from build123d import *

# Parameters (mm, degrees)
SKETCH1_W           = 225.425
SKETCH1_H           = 196.85
SKETCH1_R           = 2.5527
BOSS_EXTRUDE1_DEPTH = 3.175
FILLET1_R           = 6.35
SKETCH2_W           = 22.86
SKETCH2_H           = 31.75
CUT_EXTRUDE1_DEPTH  = 300.293223695
FILLET2_R           = 6.35
BOSS_EXTRUDE2_DEPTH = 3.175
FILLET3_R           = 6.35
SKETCH4_R           = 2.4892
CUT_EXTRUDE2_DEPTH  = 520.25515638
CUT_EXTRUDE3_DEPTH  = 520.25515638
FILLET4_R           = 12.7
FILLET5_R           = 12.7
CUT_EXTRUDE4_DEPTH  = 520.25515638
FILLET6_R           = 12.7


with BuildPart() as part:
    # Sketch1 → Boss-Extrude1 (new body)
    with BuildSketch(Plane(origin=(0, 0, 0), x_dir=(1, 0, 0), z_dir=(0, 1, 0))):
        with Locations((112.7125, 98.425)):
            Rectangle(SKETCH1_W, SKETCH1_H)
        with Locations(Location((4.7625, 187.325, 0), (0, 0, 270))):
            Circle(SKETCH1_R, mode=Mode.SUBTRACT)
        with Locations(Location((4.7625, 174.625, 0), (0, 0, 270))):
            Circle(SKETCH1_R, mode=Mode.SUBTRACT)
        with Locations(Location((4.7625, 161.925, 0), (0, 0, 270))):
            Circle(SKETCH1_R, mode=Mode.SUBTRACT)
        with Locations(Location((4.7625, 149.225, 0), (0, 0, 270))):
            Circle(SKETCH1_R, mode=Mode.SUBTRACT)
        with Locations(Location((4.7625, 136.525, 0), (0, 0, 270))):
            Circle(SKETCH1_R, mode=Mode.SUBTRACT)
        with Locations(Location((4.7625, 123.825, 0), (0, 0, 270))):
            Circle(SKETCH1_R, mode=Mode.SUBTRACT)
        with Locations(Location((220.6625, 123.825, 0), (0, 0, 90))):
            Circle(SKETCH1_R, mode=Mode.SUBTRACT)
        with Locations(Location((220.6625, 136.525, 0), (0, 0, 90))):
            Circle(SKETCH1_R, mode=Mode.SUBTRACT)
        with Locations(Location((220.6625, 149.225, 0), (0, 0, 90))):
            Circle(SKETCH1_R, mode=Mode.SUBTRACT)
        with Locations(Location((220.6625, 161.925, 0), (0, 0, 90))):
            Circle(SKETCH1_R, mode=Mode.SUBTRACT)
        with Locations(Location((220.6625, 174.625, 0), (0, 0, 90))):
            Circle(SKETCH1_R, mode=Mode.SUBTRACT)
        with Locations(Location((220.6625, 187.325, 0), (0, 0, 90))):
            Circle(SKETCH1_R, mode=Mode.SUBTRACT)
        with Locations(Location((4.7625, 111.125, 0), (0, 0, 270))):
            Circle(SKETCH1_R, mode=Mode.SUBTRACT)
        with Locations(Location((4.7625, 98.425, 0), (0, 0, 270))):
            Circle(SKETCH1_R, mode=Mode.SUBTRACT)
        with Locations(Location((4.7625, 85.725, 0), (0, 0, 270))):
            Circle(SKETCH1_R, mode=Mode.SUBTRACT)
        with Locations(Location((4.7625, 73.025, 0), (0, 0, 270))):
            Circle(SKETCH1_R, mode=Mode.SUBTRACT)
        with Locations(Location((4.7625, 60.325, 0), (0, 0, 270))):
            Circle(SKETCH1_R, mode=Mode.SUBTRACT)
        with Locations(Location((4.7625, 47.625, 0), (0, 0, 270))):
            Circle(SKETCH1_R, mode=Mode.SUBTRACT)
        with Locations(Location((4.7625, 34.925, 0), (0, 0, 270))):
            Circle(SKETCH1_R, mode=Mode.SUBTRACT)
        with Locations(Location((4.7625, 22.225, 0), (0, 0, 270))):
            Circle(SKETCH1_R, mode=Mode.SUBTRACT)
        with Locations(Location((4.7625, 9.525, 0), (0, 0, 270))):
            Circle(SKETCH1_R, mode=Mode.SUBTRACT)
        with Locations(Location((220.6625, 111.125, 0), (0, 0, 90))):
            Circle(SKETCH1_R, mode=Mode.SUBTRACT)
        with Locations(Location((220.6625, 98.425, 0), (0, 0, 90))):
            Circle(SKETCH1_R, mode=Mode.SUBTRACT)
        with Locations(Location((220.6625, 85.725, 0), (0, 0, 90))):
            Circle(SKETCH1_R, mode=Mode.SUBTRACT)
        with Locations(Location((220.6625, 73.025, 0), (0, 0, 90))):
            Circle(SKETCH1_R, mode=Mode.SUBTRACT)
        with Locations(Location((220.6625, 60.325, 0), (0, 0, 90))):
            Circle(SKETCH1_R, mode=Mode.SUBTRACT)
        with Locations(Location((220.6625, 47.625, 0), (0, 0, 90))):
            Circle(SKETCH1_R, mode=Mode.SUBTRACT)
        with Locations(Location((220.6625, 34.925, 0), (0, 0, 90))):
            Circle(SKETCH1_R, mode=Mode.SUBTRACT)
        with Locations(Location((220.6625, 22.225, 0), (0, 0, 90))):
            Circle(SKETCH1_R, mode=Mode.SUBTRACT)
        with Locations(Location((220.6625, 9.525, 0), (0, 0, 90))):
            Circle(SKETCH1_R, mode=Mode.SUBTRACT)
    extrude(amount=BOSS_EXTRUDE1_DEPTH)

    # Fillet1
    fillet1_edges = [part.edges().sort_by_distance(p)[0] for p in [
        (0, 1.5875, -196.85),
        (225.425, 1.5875, -196.85),
        (225.425, 1.5875, 0),
        (0, 1.5875, 0),
    ]]
    fillet(fillet1_edges, radius=FILLET1_R)

    # Sketch2 → Cut-Extrude1 (cut, through all)
    with BuildSketch(Plane(origin=(0, 3.175, 0), x_dir=(1, 0, 0), z_dir=(0, 1, 0))):
        with Locations((30.48, 180.975)):
            Rectangle(SKETCH2_W, SKETCH2_H)
        with Locations((194.945, 180.975)):
            Rectangle(SKETCH2_W, SKETCH2_H)
    extrude(amount=-CUT_EXTRUDE1_DEPTH, mode=Mode.SUBTRACT)

    # Fillet2
    fillet2_edges = [part.edges().sort_by_distance(p)[0] for p in [
        (19.05, 1.5875, -165.1),
        (19.05, 1.5875, -196.85),
        (41.91, 1.5875, -196.85),
        (41.91, 1.5875, -165.1),
        (183.515, 1.5875, -196.85),
        (206.375, 1.5875, -196.85),
        (206.375, 1.5875, -165.1),
        (183.515, 1.5875, -165.1),
    ]]
    fillet(fillet2_edges, radius=FILLET2_R)

    # Sketch3 → Boss-Extrude2 (add)
    with BuildSketch(Plane(origin=(0, 3.175, 0), x_dir=(1, 0, 0), z_dir=(0, 1, 0))):
        with BuildLine():
            ThreePointArc((0, 6.35), (1.859871939, 1.859871939), (6.35, 0))
            Line((6.35, 0), (-222.25, 0))
            Line((-222.25, 0), (-222.25, 263.064500032))
            Line((-222.25, 263.064500032), (-166.6875, 263.064500032))
            Line((-166.6875, 263.064500032), (-166.6875, 220.934871939))
            Line((-166.6875, 220.934871939), (6.35, 196.85))
            ThreePointArc((6.35, 196.85), (1.859871939, 194.990128061), (0, 190.5))
            Line((0, 190.5), (0, 6.35))
        make_face()
        with BuildLine():
            Line((392.1125, 220.934871939), (219.075, 196.85))
            ThreePointArc((219.075, 196.85), (223.565128061, 194.990128061), (225.425, 190.5))
            Line((225.425, 190.5), (225.425, 6.35))
            ThreePointArc((225.425, 6.35), (223.565128061, 1.859871939), (219.075, 0))
            Line((219.075, 0), (447.675, 0))
            Line((447.675, 0), (447.675, 263.064500032))
            Line((447.675, 263.064500032), (392.1125, 263.064500032))
            Line((392.1125, 263.064500032), (392.1125, 220.934871939))
        make_face()
    extrude(amount=-BOSS_EXTRUDE2_DEPTH)

    # Fillet3
    fillet3_edges = [part.edges().sort_by_distance(p)[0] for p in [
        (219.075, 1.5875, -196.85),
        (6.35, 1.5875, -196.85),
        (-222.25, 1.5875, 0),
        (-222.25, 1.5875, -263.064500032),
        (-166.6875, 1.5875, -263.064500032),
        (-166.6875, 1.5875, -220.934871939),
        (447.675, 1.5875, 0),
        (447.675, 1.5875, -263.064500032),
        (392.1125, 1.5875, -263.064500032),
        (392.1125, 1.5875, -220.934871939),
    ]]
    fillet(fillet3_edges, radius=FILLET3_R)

    # Sketch4 → Cut-Extrude2 (cut, through all)
    with BuildSketch(Plane(origin=(0, 3.175, 0), x_dir=(1, 0, 0), z_dir=(0, 1, 0))):
        with Locations(Location((-211.1375, 256.714500032, 0), (0, 0, 270))):
            Circle(SKETCH4_R)
        with Locations((-223.8375, 256.714500032)):
            Circle(SKETCH4_R)
        with Locations(Location((-198.4375, 256.714500032, 0), (0, 0, 270))):
            Circle(SKETCH4_R)
        with Locations(Location((-185.7375, 256.714500032, 0), (0, 0, 270))):
            Circle(SKETCH4_R)
        with Locations(Location((411.1625, 256.714500032, 0), (0, 0, 270))):
            Circle(SKETCH4_R)
        with Locations(Location((423.8625, 256.714500032, 0), (0, 0, 270))):
            Circle(SKETCH4_R)
        with Locations(Location((436.5625, 256.714500032, 0), (0, 0, 270))):
            Circle(SKETCH4_R)
        with Locations((449.2625, 256.714500032)):
            Circle(SKETCH4_R)
    extrude(amount=-CUT_EXTRUDE2_DEPTH, mode=Mode.SUBTRACT)

    # Sketch5 → Cut-Extrude3 (cut, through all)
    with BuildSketch(Plane(origin=(0, 3.175, 0), x_dir=(1, 0, 0), z_dir=(0, 1, 0))):
        with BuildLine():
            Line((-196.85, 201.06223924), (-166.6875, 226.46223924))
            Line((-166.6875, 226.46223924), (-166.6875, 256.714500032))
            ThreePointArc((-166.6875, 256.714500032), (-168.547371939, 261.204628093), (-173.0375, 263.064500032))
            Line((-173.0375, 263.064500032), (-215.9, 263.064500032))
            ThreePointArc((-215.9, 263.064500032), (-219.742708963, 261.769802973), (-222.01844344, 258.413661552))
            ThreePointArc((-222.01844344, 258.413661552), (-221.353386843, 256.55544512), (-222.25, 254.797220608))
            Line((-222.25, 254.797220608), (-222.25, 161.464500032))
            Line((-222.25, 161.464500032), (-196.85, 161.464500032))
            Line((-196.85, 161.464500032), (-196.85, 201.06223924))
        make_face()
    extrude(amount=-CUT_EXTRUDE3_DEPTH, mode=Mode.SUBTRACT)

    # Fillet4
    fillet4_edges = [part.edges().sort_by_distance(p)[0] for p in [
        (-166.6875, 1.5875, -226.46223924),
    ]]
    fillet(fillet4_edges, radius=FILLET4_R)

    # Fillet5
    # the kernel refuses this fillet: 12.7 mm, written as the material it adds along each edge
    with BuildSketch(Plane(origin=(-196.85, 3.175, -161.464500032), x_dir=(0, 0, -1), z_dir=(0, -1, 0))) as fillet5_piece_1:
        with BuildLine():
            CenterArc((FILLET5_R, -FILLET5_R), FILLET5_R, 90, 90)
            Line((0, -FILLET5_R), (0, 0))
            Line((0, 0), (FILLET5_R, 0))
        make_face()
    extrude(amount=3.175)
    # the kernel refuses this fillet: 12.7 mm, written as the material it takes off along each edge
    with BuildSketch(Plane(origin=(-196.85, 17.946244164, -201.06223924), x_dir=(0.7649111981170551, 0, -0.6441357457827745), z_dir=(0, -1, 0))) as fillet5_2_piece_1:
        with BuildLine():
            CenterArc((FILLET5_R * 0.465236036671, FILLET5_R), FILLET5_R, 220.100907546, 49.899092454)
            Line((-FILLET5_R * 0.299675161446, FILLET5_R * 0.355864254217), (0, 0))
            Line((0, 0), (FILLET5_R * 0.465236036671, 0))
        make_face()
    extrude(amount=32.717488329, mode=Mode.SUBTRACT)
    with BuildSketch(Plane(origin=(447.675, -8.095541775, -254.797220608), x_dir=(0, 0, 1), z_dir=(0, 1, 0))) as fillet5_2_piece_2:
        with BuildLine():
            CenterArc((3.23821671, -12.7), FILLET5_R, 90, 19.84145254)
            ThreePointArc((-1.072398787, -0.753929766), (-0.485677324, -0.448828084), (0, 0))
            Line((0, 0), (3.23821671, 0))
        make_face()
    extrude(amount=19.366083551, mode=Mode.SUBTRACT)
    with BuildSketch(Plane(origin=(447.44344344, 35.300659999, -258.413661552), x_dir=(-0.15933009904397483, 0, 0.987225364108235), z_dir=(0, -1, 0))) as fillet5_2_piece_3:
        with BuildLine():
            CenterArc((9.854968596, 10.543603817), FILLET5_R, 170.831985075, 65.287819707)
            Line((-2.682793528, 12.567096075), (-3.936569741, 12.7694453))
            ThreePointArc((-3.936569741, 12.7694453), (-4.870349725, 6.983650334), (-0.53046151, -1.153910996))
            Line((-0.53046151, -1.153910996), (0.707971882, -1.054360382))
            ThreePointArc((0.707971882, -1.054360382), (1.387624889, -0.847346348), (2.067277895, -1.054360382))
            Line((2.067277895, -1.054360382), (2.775249777, 0))
        make_face()
    extrude(amount=67.426319998, mode=Mode.SUBTRACT)
    with BuildSketch(Plane(origin=(-222.25, 34.925, -161.464500032), x_dir=(1, 0, 0), z_dir=(0, -1, 0))) as fillet5_2_piece_4:
        with BuildLine():
            CenterArc((FILLET5_R, FILLET5_R), FILLET5_R, 180, 90)
            Line((0, FILLET5_R), (0, 0))
            Line((0, 0), (FILLET5_R, 0))
        make_face()
    extrude(amount=66.675, mode=Mode.SUBTRACT)

    # Sketch6 → Cut-Extrude4 (cut, through all)
    with BuildSketch(Plane(origin=(0, 3.175, 0), x_dir=(1, 0, 0), z_dir=(0, 1, 0))):
        with BuildLine():
            ThreePointArc((392.1125, 226.46223924), (390.552142427, 222.293087597), (386.637909316, 220.172870549))
            Line((386.637909316, 220.172870549), (447.675, 220.172870549))
            Line((447.675, 220.172870549), (447.675, 251.559003898))
            ThreePointArc((447.675, 251.559003898), (447.494110467, 253.694858088), (446.956594784, 255.769869181))
            ThreePointArc((446.956594784, 255.769869181), (442.270283564, 261.086864235), (435.464337201, 263.064500032))
            Line((435.464337201, 263.064500032), (398.4625, 263.064500032))
            ThreePointArc((398.4625, 263.064500032), (393.972371939, 261.204628093), (392.1125, 256.714500032))
            Line((392.1125, 256.714500032), (392.1125, 226.46223924))
        make_face()
    extrude(amount=-CUT_EXTRUDE4_DEPTH, mode=Mode.SUBTRACT)

    # Fillet6
    fillet6_edges = [part.edges().sort_by_distance(p)[0] for p in [
        (386.637909316, 1.5875, -220.172870549),
        (447.675, 1.5875, -220.172870549),
    ]]
    fillet(fillet6_edges, radius=FILLET6_R)


solid = part.part
Geometry: final body of the model. Coordinates: model frame, mm. A direction names the side the tool comes from. Give positions to 0.01 mm unless a question says otherwise; leave off trailing zeros. Loops run counter-clockwise (first coordinate to the right, second up) from the corner with the lowest first, then second, coordinate; pieces in that order, holes last. Notation, with made-up numbers: (71, 6) -> (90, 6) arc R11 cw to (90, 17) -> close; hole circle Ø4 at (59.5, -22.75). An arc over 180 degrees is marked (long way). Put each result on its own line as item: value.
1. Cut plane A-A (x = 145). Return the cut outline in (y, z) (3 decimals).
Taken from the geometry:
outline: (0, -196.85) -> (3.175, -196.85) -> (3.175, 0) -> (0, 0) -> close
2. Cut plane B-B (y = 2). Count the separate pieces of the cut face and the enclosed holes in it, plus the area to 3 significant figures.
Taken from the geometry:
separate pieces: 1
enclosed holes: 30
area: 135,000 mm2
3. Pin query (flat end, axial travel): P1, Ø4, axis at x = 220.66, z = -136.52, coming from the +Y side; P2, Ø1, axis at x = 368.5, y = 3, coming from the -Z side; P3, Ø1, axis at x = 413.5, y = 1, coming from the -Z side; P4, Ø1.6, axis at y = 1.5, z = -181, coming from the -X side. Return the tip coordinate at first contact, or that it passes through.
Taken from the geometry:
P1: passes through
P2: stops at z = -217.72
P3: stops at z = -220.17
P4: stops at x = -196.85
4. Ray query, line 1 along X through (y, z) = (2.8, -187.5) (3 decimals); line 2 along X through (y, z) = (0.75, -35) (3 decimals); line 3 along X through (y, z) = (1.1, -11.5) (3 decimals). Return the intervals inside material, ascending. Write a range as [from, to].
Taken from the geometry:
line 1: x = [-196.85, 2.216], [7.309, 19.05], [41.91, 183.515], [206.375, 218.116], [223.209, 447.675]
line 2: x = [-222.25, 2.211], [7.314, 218.111], [223.214, 447.675]
line 3: x = [-222.25, 3.145], [6.38, 219.045], [222.28, 447.675]
5. Set-up query: faces 1 (the flat face through (303.802, 1.61, -208.643)), 2 (the flat face through (117, 3.175, -112)). Return all of +Z, -Z, +X, -X, +Y, -Y with unobstructed straight access to the full face (end or side cutting, diameter ignored); none if empty.
Taken from the geometry:
face 1: -Z, +Y, -Y
face 2: +Z, -Z, +X, -X, +Y
6. Cut plane C-C (x = 255). Return the cut outline in (y, z) (3 decimals), plus the area to 3 significant figures.
Taken from the geometry:
outline: (0, -201.85) -> (3.175, -201.85) -> (3.175, 0) -> (0, 0) -> close
area: 641 mm2
